Input: part model. Units: mm. Frame: model coordinates. Face numbers are marked on the shaded views. A direction names the side the tool comes from. Give positions to 0.01 mm unless a question says otherwise; leave off trailing zeros. Loops run counter-clockwise (first coordinate to the right, second up) from the corner with the lowest first, then second, coordinate; pieces in that order, holes last. Notation, with made-up numbers: M -31,34.25 L -14,34.25 A24 cw -14,58.25 Z; hole C 21.25,72.25 d9. An arc over 180 degrees is marked long. Answer as a JSON object with one key per item and string values. Group by question number.
1) Ray query, L1, parallel to Y at x = -5.2, z = -70; L2, parallel to Z at x = -6.7, y = 3.6; L3, parallel to X at y = 14.5, z = -6. Return the intervals inside material, ascending.
2) Section query B-B on z = -32.5. Return loops of the section in (x, y) (3 decimals), plus the area to 3 significant figures.
3) First-contact query: P1, Ø5, axis at y = 3, z = -8, coming from the +X side; P2, Ø8.5, axis at y = -1, z = -27.5, coming from the +X side; P3, Ø3.5, axis at y = 13.6, z = -70, coming from the -X side. Flat tips, straight axial feed; report the tip coordinate or a pass-through.
4) Access query for the marked faces 1, 2 and 3. Directions: +Z, -Z, +X, -X, +Y, -Y. A direction counts if a zero-diameter tool reaches every point of the face in a straight line with its end or side. Return the directions, or none.
5) Section query A-A on z = -70. Count the separate pieces of the cut face and the enclosed holes in it, plus the area to 3 significant figures.
6) Section query C-C on z = -7. Return loops of the section in (x, y) (3 decimals).
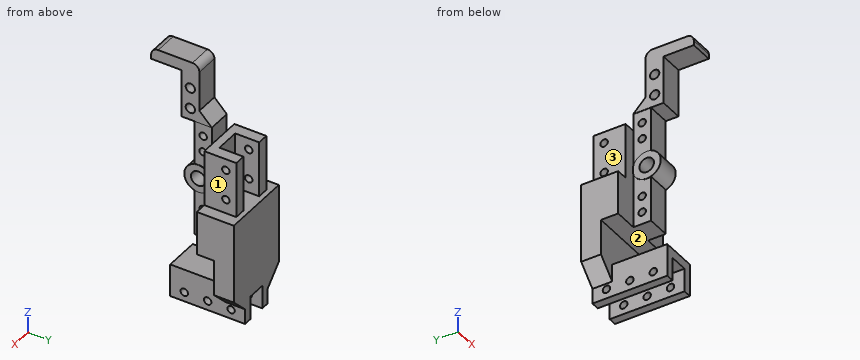
from build123d import *

# Parameters (mm, degrees)
SKETCH_2_W               = 50
SKETCH_2_H               = 7.55
SKETCH_2_R               = 1.6
EXTRUDE_1_DEPTH          = 4.9
SKETCH_3_W               = 23.885574904
SKETCH_3_H               = 13.680093874
SKETCH_3_R               = 1.6
EXTRUDE_2_DEPTH          = 10
SKETCH_4_W               = 10.5
SKETCH_4_H               = 10.264550668
CUT_EXTRUDE_1_DEPTH      = 48.143107127
SKETCH_6_W               = 14
SKETCH_6_H               = 32
SKETCH_6_R               = 1.6
EXTRUDE_4_DEPTH          = 7.5
SKETCH_7_W               = 8
SKETCH_7_H               = 32
CUT_EXTRUDE_2_DEPTH      = 10
EXTRUDE_5_DEPTH          = 15
CHAMFER_1_SIZE           = 7.5
SKETCH_10_R              = 2
EXTRUDE_6_DEPTH          = 5
FILLET_1_R               = 3
SKETCH_11_R              = 6
SKETCH_11_R_2            = 3.125
EXTRUDE_7_DEPTH          = 5
CUT_EXTRUDE_3_DEPTH      = 79.685454984
CUT_EXTRUDE_3_DEPTH_BACK = 79.685454984
SKETCH_12_R              = 3.125


with BuildPart() as part:
    # Sketch 2 → Extrude 1 (new, symmetric)
    with BuildSketch(Plane(origin=(0, 0, 0), x_dir=(0, 0, -1), z_dir=(1, 0, 0))):
        with Locations((19.75, 0)):
            Rectangle(SKETCH_2_W, SKETCH_2_H)
        Circle(SKETCH_2_R, mode=Mode.SUBTRACT)
        with Locations((7, 0)):
            Circle(SKETCH_2_R, mode=Mode.SUBTRACT)
        with Locations((32.5, 0)):
            Circle(SKETCH_2_R, mode=Mode.SUBTRACT)
        with Locations((39.5, 0)):
            Circle(SKETCH_2_R, mode=Mode.SUBTRACT)
    extrude(amount=EXTRUDE_1_DEPTH, both=True)

    # Sketch 3 → Extrude 2 (add, symmetric)
    with BuildSketch(Plane(origin=(0, 0, 0), x_dir=(0, 0, -1), z_dir=(1, 0, 0))):
        with Locations((14.057212548, 10.615046937)):
            Rectangle(SKETCH_3_W, SKETCH_3_H)
        with Locations((7, 13)):
            Circle(SKETCH_3_R, mode=Mode.SUBTRACT)
        with Locations((20, 13)):
            Circle(SKETCH_3_R, mode=Mode.SUBTRACT)
    extrude(amount=EXTRUDE_2_DEPTH, both=True)

    # Sketch 4 → Cut-Extrude 1 (cut, through all)
    with BuildSketch(Plane.XY.offset(-2.114425096)):
        with Locations((0, 12.32281854)):
            Rectangle(SKETCH_4_W, SKETCH_4_H)
    extrude(amount=-CUT_EXTRUDE_1_DEPTH, mode=Mode.SUBTRACT)



with BuildPart() as body_2:
    # Sketch 6 → Extrude 4 (new, symmetric)
    with BuildSketch(Plane(origin=(0, 0, 0), x_dir=(0, 0, -1), z_dir=(1, 0, 0))):
        with Locations((67, 3.6)):
            Rectangle(SKETCH_6_W, SKETCH_6_H)
        with Locations((70, 3.6)):
            Circle(SKETCH_6_R, mode=Mode.SUBTRACT)
        with Locations((70, 13.6)):
            Circle(SKETCH_6_R, mode=Mode.SUBTRACT)
        with Locations((70, -6.4)):
            Circle(SKETCH_6_R, mode=Mode.SUBTRACT)
    extrude(amount=EXTRUDE_4_DEPTH, both=True)

    # Sketch 7 → Cut-Extrude 2 (cut)
    with BuildSketch(Plane.XY.offset(-74)):
        with Locations((0, 3.6)):
            Rectangle(SKETCH_7_W, SKETCH_7_H)
    extrude(amount=CUT_EXTRUDE_2_DEPTH, mode=Mode.SUBTRACT)


with BuildPart() as part_1:
    add(part.part)

    add(body_2.part)  # Extrude 5 merges body 2
    # Sketch 8 → Extrude 5 (add, symmetric)
    with BuildSketch(Plane(origin=(0, 0, 0), x_dir=(0, 0, -1), z_dir=(1, 0, 0))):
        Polygon((60, 19.6), (26, 19.6), (26, 11.139938787), (26, 3.775), (44.75, 3.775), (44.75, 11.139938787), (60, 11.139938787), align=None)
    extrude(amount=EXTRUDE_5_DEPTH, both=True)

    # Chamfer 1
    chamfer_1_edges = [part_1.edges().sort_by_distance(p)[0] for p in [
        (-7.5, 15.369969393, -60),
        (7.5, 15.369969393, -60),
    ]]
    chamfer(chamfer_1_edges, length=CHAMFER_1_SIZE - 0.0001)  # a hair under: the kernel refuses the full size

    # Sketch 10 → Extrude 6 (add, symmetric)
    with BuildSketch(Plane(origin=(0, 0, 0), x_dir=(0, 0, -1), z_dir=(1, 0, 0))):
        Polygon((-5.25, 3.775), (-5.25, -9.176683543), (-25.75, -9.176683543), (-25.75, -22.144995508), (-30.75, -22.144995508), (-30.75, -1.524124881), (-10.688710914, -1.524124881), align=None)
        with Locations((-10.25, -5.401683543)):
            Circle(SKETCH_10_R, mode=Mode.SUBTRACT)
        with Locations((-19.25, -5.401683543)):
            Circle(SKETCH_10_R, mode=Mode.SUBTRACT)
    extrude(amount=EXTRUDE_6_DEPTH, both=True)

    # Fillet 1
    fillet_1_edges = [part_1.edges().sort_by_distance(p)[0] for p in [
        (0, -1.524124881, 30.75),
        (0, -22.144995508, 30.75),
    ]]
    fillet(fillet_1_edges, radius=FILLET_1_R)

    # Sketch 11 → Extrude 7 (add, symmetric)
    with BuildSketch(Plane(origin=(0, 0, 0), x_dir=(0, 0, -1), z_dir=(1, 0, 0))):
        with Locations((19.487465682, -2)):
            Circle(SKETCH_11_R)
        with Locations((19.487465682, -2)):
            Circle(SKETCH_11_R_2, mode=Mode.SUBTRACT)
    extrude(amount=EXTRUDE_7_DEPTH, both=True)

    # Sketch 12 → Cut-Extrude 3 (cut, two sides: drawn at the far end of the back side and taken through both)
    with BuildSketch(Plane(origin=(0, 0, 0), x_dir=(0, 0, -1), z_dir=(1, 0, 0)).offset(-CUT_EXTRUDE_3_DEPTH_BACK)):
        with Locations((19.487465682, -2)):
            Circle(SKETCH_12_R)
    extrude(amount=CUT_EXTRUDE_3_DEPTH + CUT_EXTRUDE_3_DEPTH_BACK, mode=Mode.SUBTRACT)


solid = part_1.part
Output:
{
 "1": {"L1": "y = -12.4 to -8, -4.8 to 2, 5.2 to 12, 15.2 to 19.6", "L2": "z = -74 to -71.6, -68.4 to -60", "L3": "x = -10 to -5.25, 5.25 to 10"},
 "2": {"outline": "M -15,3.775 L -4.9,3.775 L -4.9,1.6 L 4.9,1.6 L 4.9,3.775 L 15,3.775 L 15,19.6 L -15,19.6 Z; M -4.9,-3.775 L 4.9,-3.775 L 4.9,-1.6 L -4.9,-1.6 Z", "area": "517 mm^2"},
 "3": {"P1": "stops at x = 10", "P2": "stops at x = 5", "P3": "stops at x = -7.5"},
 "4": {"face 1": "+Z, +X, +Y, -Y", "face 2": "+X, -X, -Y", "face 3": "+Z, -X, +Y, -Y"},
 "5": {"separate pieces": "8", "enclosed holes": "0", "area": "157 mm^2"},
 "6": {"outline": "M -10,3.775 L -4.9,3.775 L -4.9,1.6 L 4.9,1.6 L 4.9,3.775 L 10,3.775 L 10,11.4 L 5.25,11.4 L 5.25,7.191 L -5.25,7.191 L -5.25,11.4 L -10,11.4 Z; M -10,14.6 L -5.25,14.6 L -5.25,17.455 L -10,17.455 Z; M -4.9,-3.775 L 4.9,-3.775 L 4.9,-1.6 L -4.9,-1.6 Z; M 5.25,14.6 L 10,14.6 L 10,17.455 L 5.25,17.455 Z"}
}
